Source: three-view drawing plus pictorial views. Frame: mm from the lowest corner of the part. A direction names the side the tool comes from. Coordinates: 2 decimals unless noted, no trailing zeros. Loops run counter-clockwise (first coordinate to the right, second up) from the corner with the lowest first, then second, coordinate; pieces in that order, holes last. Notation, with made-up numbers: M -27,4.5 L 21,4.5 A35 ccw 21,37.5 Z; hole C 85.5,-9.5 d1. An arc over 180 degrees is marked long. Write each question's results on one line, items separated by ' | '. Start each with the question number.
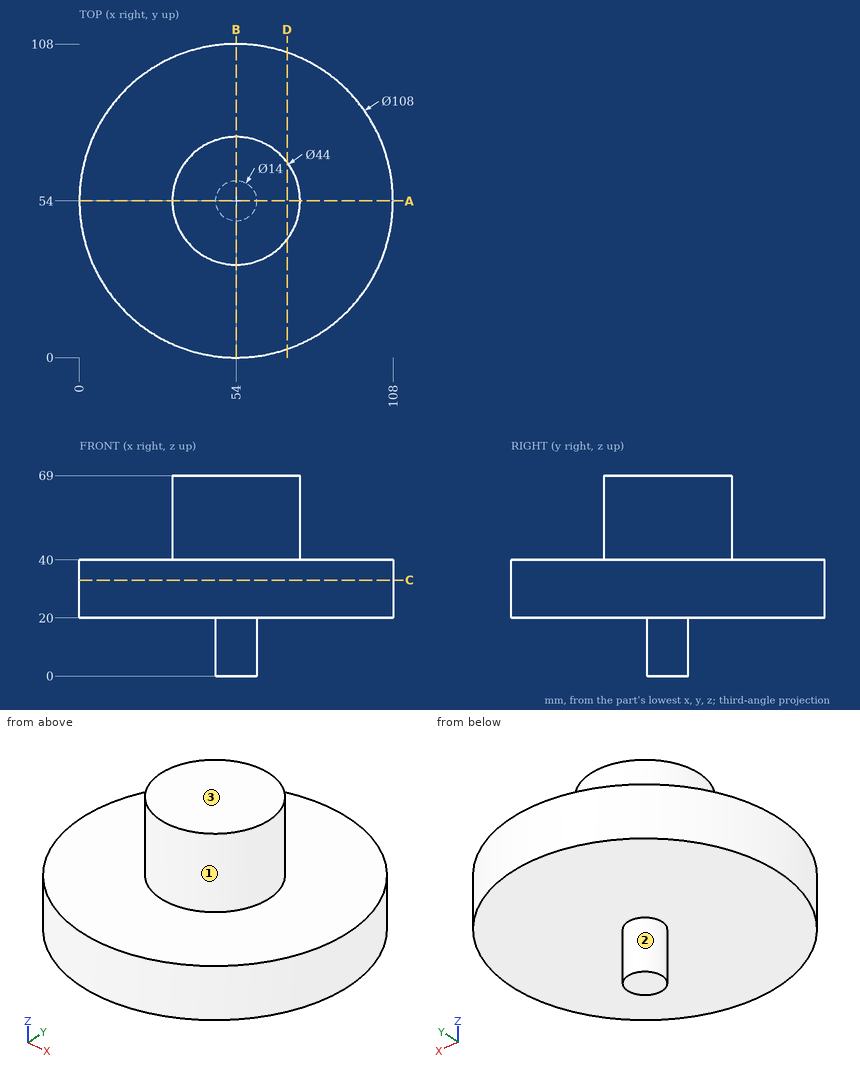
Item 1: Contact query for flat-ended pins moving along their axis: P1, Ø3, axis at x = 67, y = 82, coming from the +Z side; P2, Ø12, axis at x = 61.5, z = 55, coming from the +Y side; P3, Ø1, axis at x = 66.5, z = 53, coming from the +Y side. Output: stop coordinate, or through.
Item 2: Ray query, L1, parallel to Z at x = 42, y = 27; L2, parallel to Z at x = 61, y = 73; L3, parallel to X at y = 67, z = 43.5. Return the intervals inside material, ascending. Write a range as [from, to].
Item 3: Section C-C, the plane z = 33. Return loops of the section in (x, y).
Item 4: Section D-D, the plane x = 71.5. Return loops of the section in (y, z).
Item 5: Section A-A, the plane y = 54. Return loops of the section in (x, z).
Item 6: Set-up query: the marked faces 1, 2 and 3. Return all of +Z, -Z, +X, -X, +Y, -Y with unobstructed straight access to the full face (end or side cutting, diameter ignored); none if empty.
Solutions:
1) P1: stops at z = 40 | P2: stops at y = 75.95 | P3: stops at y = 72.44
2) L1: z = [20, 40] | L2: z = [20, 69] | L3: x = [36.25, 71.75]
3) outline: C 54,54 d108
4) outline: M 2.91,20 L 105.09,20 L 105.09,40 L 67.33,40 L 67.33,69 L 40.67,69 L 40.67,40 L 2.91,40 Z
5) outline: M 0,20 L 47,20 L 47,0 L 61,0 L 61,20 L 108,20 L 108,40 L 76,40 L 76,69 L 32,69 L 32,40 L 0,40 Z
6) face 1: +Z | face 2: -Z | face 3: +Z, +X, -X, +Y, -Y
